Autodesk Inventor part; units mm, degrees
ref_plane "YZ Plane" through (0, 0, 0) normal (1, 0, 0) x (0, 1, 0)
ref_plane "XZ Plane" through (0, 0, 0) normal (0, 1, 0) x (-1, 0, 0)
ref_plane "XY Plane" through (0, 0, 0) normal (0, 0, 1) x (1, 0, 0)
sketch "Szkic1" plane through (0, 0, 0) normal (0, 1, 0) x (-1, 0, 0)
  line L0 (-25, 25) -> (25, 25)
  line L1 (25, 25) -> (25, -25)
  line L2 (25, -25) -> (-25, -25)
  line L3 (-25, -25) -> (-25, 25)
  line L4 (-25, 25) -> (25, -25) construction
  line L5 (25, 25) -> (-25, -25) construction
  point P0 (0, 0)
  dimension "d0" = 50
  dimension "d1" = 50
extrude "Wyciągnięcie proste1" add sketch "Szkic1" along normal blind 30
sketch "Szkic2" plane through (0, 30, 0) normal (0, 1, 0) x (1, 0, 0)
  circle A0 centre (0, 0) radius 12.5
  dimension "d4" = 25
extrude "Wyciągnięcie proste2" cut sketch "Szkic2" against normal up to next
sketch "Szkic3" plane through (0, 30, 0) normal (0, 1, 0) x (1, 0, 0)
  circle A0 centre (0, 0) radius 22.5
  dimension "d7" = 45
extrude "Wyciągnięcie proste3" cut sketch "Szkic3" against normal blind 15
sketch "Szkic4" plane through (0, 15, 0) normal (0, 1, 0) x (1, 0, 0)
  circle A0 centre (0, 0) radius 12.25
  circle A1 centre (0, 0) radius 21
  circle A2 centre (-17, 0) radius 2.5
  circle A3 centre (-8.5, -14.7224) radius 2.5
  circle A4 centre (8.5, -14.7224) radius 2.5
  circle A5 centre (17, 0) radius 2.5
  circle A6 centre (8.5, 14.7224) radius 2.5
  circle A7 centre (-8.5, 14.7224) radius 2.5
  dimension "d11" = 5
  dimension "d14" = 360
  dimension "d36" = 17
extrude "Wyciągnięcie proste4" cut sketch "Szkic4" against normal blind 10 contours A2 | A3 | A4 | A5 | A6 | A7
thread "Gwint1"
thread "Gwint2"
thread "Gwint3"
thread "Gwint4"
thread "Gwint5"
thread "Gwint6"
properties part number "Obudowa nakrętki trapezowej fi 10"
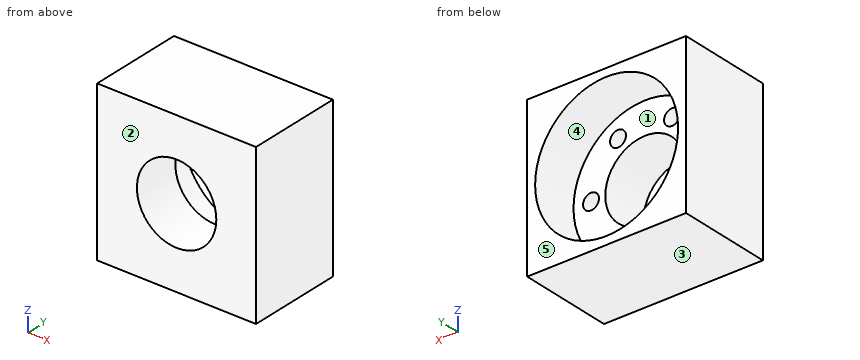
Read the model definition and answer for the solid it produces. Units are mm, in the model's axes. Face numbers are marked on the shaded views. A direction names the side the tool comes from. Give positions to 0.01 mm unless a question says otherwise; leave off trailing zeros. Write each loop counter-clockwise with the first axis right and the second up, starting at its lowest first coordinate (ties: lowest second). Pieces come first, ordered by that corner, then holes. Notation, with made-up numbers: M 43.25,18 L 70.25,18 A18 ccw 70.25,23 Z; hole C -23,5.25 d2. An arc over 180 degrees is marked long. One line per item, written item: value. Start each with the question number.
(1) Find section B-B (z = 0). Determine the outline of the cut face in (x, y).
(2) Find the intervals of material crossed by line 1 (X direction, y = 6.75, z = 0); line 2 (Z direction, x = 0, y = 11); line 3 (X direction, y = 22.5, z = 0), in increasing order.
(3) Find section C-C (y = 23). Determine the outline of the cut face in (x, z).
(4) Flat-ended cylindrical pins translate along their axes: pin 1 Ø5.5 at (x, z) = (-16, 0.5) entering from +Y; pin 2 Ø1.5 at (x, z) = (9.5, -15) entering from +Y. Find the tip coordinate at first contact, or state that the pin passes through.
(5) Find section D-D (x = -17). Determine the outline of the cut face in (y, z), plus the area to 3 significant figures.
(6) Determine the mould class of the marked faces 3, 4 and 5 for opening direction Z: pulls with the +Z half, pulls with the -Z half, needs draft (parallel to the pull), parting line crosses it, or undercut.
(7) Find section A-A (x = 0). Determine the outline of the cut face in (y, z).
(8) A tool of negligible diameter and unlimited length cuts with its end or side. For the marked faces 1 and 2, from which of +Z, -Z, +X, -X, +Y, -Y can it reach the whole face along a straight path? Write none if from no direction.
Results below:
1. outline: M -25,0 L -12.5,0 L -12.5,15 L -14.5,15 L -14.5,5 L -19.5,5 L -19.5,15 L -22.5,15 L -22.5,30 L -25,30 Z; M 12.5,0 L 25,0 L 25,30 L 22.5,30 L 22.5,15 L 19.5,15 L 19.5,5 L 14.5,5 L 14.5,15 L 12.5,15 Z
2. line 1: x = -25 to -19.5, -14.5 to -12.5, 12.5 to 14.5, 19.5 to 25
2. line 2: z = -25 to -12.5, 12.5 to 25
2. line 3: x = -25 to -22.5, 22.5 to 25
3. outline: M -25,-25 L 25,-25 L 25,25 L -25,25 Z; hole C 0,0 d45
4. pin 1: stops at y = 15
4. pin 2: stops at y = 5
5. outline: M 0,-25 L 30,-25 L 30,-14.74 L 15,-14.74 L 15,-2.5 L 5,-2.5 L 5,2.5 L 15,2.5 L 15,14.74 L 30,14.74 L 30,25 L 0,25 Z
5. area: 1,010 mm^2
6. face 3: pulls with the -Z half
6. face 4: undercut
6. face 5: needs draft
7. outline: M 0,-25 L 30,-25 L 30,-22.5 L 15,-22.5 L 15,-12.5 L 0,-12.5 Z; M 0,12.5 L 15,12.5 L 15,22.5 L 30,22.5 L 30,25 L 0,25 Z
8. face 1: +Y
8. face 2: +Z, -Z, +X, -X, -Y
